from build123d import *

# Parameters (mm, degrees)
EXTRUDE_1_DEPTH     = 220
SKETCH_2_R          = 4.25
CUT_EXTRUDE_1_DEPTH = 2
SKETCH_3_R          = 2.25
CUT_EXTRUDE_2_DEPTH = 2
SKETCH_4_R          = 2.25
CUT_EXTRUDE_3_DEPTH = 2


with BuildPart() as part:
    # Эскиз1 → Бобышка-Вытянуть1 (new body)
    with BuildSketch(Plane(origin=(0, 0, 0), x_dir=(1, 0, 0), z_dir=(0, 1, 0))):
        Polygon((0, 0), (0, 20), (1, 20), (1, 1), (20, 1), (20, 0), align=None)
    extrude(amount=EXTRUDE_1_DEPTH)

    # Эскиз2 → Вырез-Вытянуть1 (cut, through all)
    with BuildSketch(Plane(origin=(1, 0, 0), x_dir=(0, 0, -1), z_dir=(1, 0, 0))):
        with Locations((10.5, 180)):
            Circle(SKETCH_2_R)
        with Locations((10.5, 120)):
            Circle(SKETCH_2_R)
        with Locations((10.5, 60)):
            Circle(SKETCH_2_R)
    extrude(amount=-CUT_EXTRUDE_1_DEPTH, mode=Mode.SUBTRACT)

    # Эскиз3 → Вырез-Вытянуть2 (cut, through all)
    with BuildSketch(Plane(origin=(1, 0, 0), x_dir=(0, 0, -1), z_dir=(1, 0, 0))):
        with Locations((10.5, 210)):
            Circle(SKETCH_3_R)
    extrude(amount=-CUT_EXTRUDE_2_DEPTH, mode=Mode.SUBTRACT)

    # Эскиз4 → Вырез-Вытянуть3 (cut, through all)
    with BuildSketch(Plane(origin=(1, 0, 0), x_dir=(0, 0, -1), z_dir=(1, 0, 0))):
        with Locations((10.5, 10)):
            Circle(SKETCH_4_R)
    extrude(amount=-CUT_EXTRUDE_3_DEPTH, mode=Mode.SUBTRACT)


solid = part.part
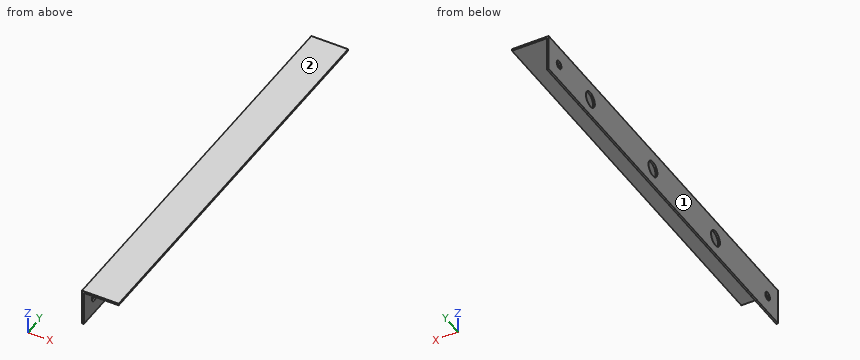
Here's how the part is built. I have some questions about the finished solid (model axes, mm). Face numbers are marked on the shaded views. Give positions to 0.01 mm unless a question says otherwise; leave off trailing zeros. Order: outer loops, then holes, each group sorted by start corner. A loop starts at its lowest first (then second) coordinate and runs counter-clockwise, first axis right, second up. Notation, with made-up numbers: M 24.25,58.5 L 35.25,58.5 A17 ccw 35.25,73.5 Z; hole C 0.5,14 d11. An arc over 180 degrees is marked long. Answer as a JSON object with one key per item and string values. Group by question number.
1) We'd pull the mould along X, two halves only. Please class the marked faces 1 and 2: pulls with the +X half, pulls with the -X half, needs draft (parallel to the pull), parting line crosses it, or undercut.
2) I'm going to push flat-ended pins straight in: pin 1 Ø1.5 at (x, y) = (14.5, 113) entering from -Z; pin 2 Ø1.5 at (y, z) = (178, -2) entering from +X. Where does each tip first touch, or does it pass through?
3) Suppose I cut it at C-C, the plane y = 10. Write out the boundary of the cut face in (x, z).
4) Suppose I cut it at A-A, the plane z = -10.5. Write out the boundary of the cut face in (x, y), plus the area to 4 significant figures.
5) Please list where these lines run through material, in increasing order: L1, parallel to Y at x = 0.6, z = -10.5; L2, parallel to Z at x = 0.75, y = 210; L3, parallel to X at y = 162.5, z = -12. Write a range as [from, to].
6) Suppose I cut it at B-B, the plane y = 180. Write out the boundary of the cut face in (x, z).
7) Suppose I cut it at D-D, the plane x = 3.5. Write out the boundary of the cut face in (y, z), plus the area to 3 significant figures.
Results found:
{
 "1": {"face 1": "pulls with the -X half", "face 2": "needs draft"},
 "2": {"pin 1": "z = -1", "pin 2": "x = 1"},
 "3": {"outline": "M 0,-20 L 1,-20 L 1,-12.75 L 0,-12.75 Z; M 0,-8.25 L 1,-8.25 L 1,-1 L 20,-1 L 20,0 L 0,0 Z"},
 "4": {"outline": "M 0,0 L 1,0 L 1,7.75 L 0,7.75 Z; M 0,12.25 L 1,12.25 L 1,55.75 L 0,55.75 Z; M 0,64.25 L 1,64.25 L 1,115.75 L 0,115.75 Z; M 0,124.25 L 1,124.25 L 1,175.75 L 0,175.75 Z; M 0,184.25 L 1,184.25 L 1,207.75 L 0,207.75 Z; M 0,212.25 L 1,212.25 L 1,220 L 0,220 Z", "area": "185.5 mm²"},
 "5": {"L1": "[0, 7.75], [12.25, 55.75], [64.25, 115.75], [124.25, 175.75], [184.25, 207.75], [212.25, 220]", "L2": "[-20, -12.75], [-8.25, 0]", "L3": "[0, 1]"},
 "6": {"outline": "M 0,-20 L 1,-20 L 1,-14.75 L 0,-14.75 Z; M 0,-6.25 L 1,-6.25 L 1,-1 L 20,-1 L 20,0 L 0,0 Z"},
 "7": {"outline": "M 0,-1 L 220,-1 L 220,0 L 0,0 Z", "area": "220 mm²"}
}
